from build123d import *

# Parameters (mm, degrees)
SKETCH1_R           = 2
BOSS_EXTRUDE2_DEPTH = 80


with BuildPart() as part:
    # Sketch1 → Boss-Extrude2 (new body)
    with BuildSketch(Plane(origin=(0, 0, 0), x_dir=(1, 0, 0), z_dir=(0, 1, 0))):
        Polygon((-12.5, 5.283121635), (-12.5, -5.283121635), (0, -12.5), (12.5, -5.283121635), (12.5, 5.283121635), (0, 12.5), align=None)
        Circle(SKETCH1_R, mode=Mode.SUBTRACT)
        with BuildLine():
            Line((-1.08, 9.382308546), (-1.08, 3.851441289))
            ThreePointArc((-1.08, 3.851441289), (-2.828427125, 2.828427125), (-3.851441289, 1.08))
            Line((-3.851441289, 1.08), (-10.34, 1.08))
            Line((-10.34, 1.08), (-10.34, 4.036045054))
            Line((-10.34, 4.036045054), (-1.08, 9.382308546))
        make_face(mode=Mode.SUBTRACT)
        with BuildLine():
            Line((1.08, 9.382308546), (1.08, 3.851441289))
            ThreePointArc((1.08, 3.851441289), (2.828427125, 2.828427125), (3.851441289, 1.08))
            Line((3.851441289, 1.08), (10.34, 1.08))
            Line((10.34, 1.08), (10.34, 4.036045054))
            Line((10.34, 4.036045054), (1.08, 9.382308546))
        make_face(mode=Mode.SUBTRACT)
        with BuildLine():
            Line((-10.34, -1.08), (-3.851441289, -1.08))
            ThreePointArc((-3.851441289, -1.08), (-2.828427125, -2.828427125), (-1.08, -3.851441289))
            Line((-1.08, -3.851441289), (-1.08, -9.382308546))
            Line((-1.08, -9.382308546), (-10.34, -4.036045054))
            Line((-10.34, -4.036045054), (-10.34, -1.08))
        make_face(mode=Mode.SUBTRACT)
        with BuildLine():
            Line((1.08, -3.851441289), (1.08, -9.382308546))
            Line((1.08, -9.382308546), (10.34, -4.036045054))
            Line((10.34, -4.036045054), (10.34, -1.08))
            Line((10.34, -1.08), (3.851441289, -1.08))
            ThreePointArc((3.851441289, -1.08), (2.828427125, -2.828427125), (1.08, -3.851441289))
        make_face(mode=Mode.SUBTRACT)
    extrude(amount=BOSS_EXTRUDE2_DEPTH)


solid = part.part
Verification items for the finished model (mm, model axes). A direction names the side the tool comes from. Give positions to 0.01 mm unless a question says otherwise; leave off trailing zeros. Write each loop counter-clockwise with the first axis right and the second up, starting at its lowest first coordinate (ties: lowest second). Pieces come first, ordered by that corner, then holes. Notation, with made-up numbers: M -38,13 L 6,13 A35 cw 6,47 Z; hole C 38.5,9 d6. An arc over 180 degrees is marked long. Write item = value, one per line.
(1) Go/stop test with flat-tipped pins: pin 1 Ø3 at (x, y) = (8.5, 22.5) entering from -Z; pin 2 Ø1.7 at (y, z) = (30, 7) entering from +X; pin 3 Ø5 at (x, y) = (-6, 43) entering from -Z; pin 4 Ø1 at (x, z) = (-4, 3.5) entering from +Y. Record where each tip stops, or that it passes through.
Found:
pin_1 = -8.46
pin_2 = 11
pin_3 = -10.48
pin_4 = through
(2) Sectioned sample at A-A (z = 0). Record the cut outline in (x, y), then the cut area to 3 significant figures.
Found:
outline = M -12.5,0 L -2,0 L -2,80 L -12.5,80 Z; M 2,0 L 12.5,0 L 12.5,80 L 2,80 Z
area = 1,680 mm2
(3) Sectioned sample at C-C (x = 5.5). Record the cut outline in (y, z), then the cut area to 3 significant figures.
Found:
outline = M 0,-9.32 L 80,-9.32 L 80,-6.83 L 0,-6.83 Z; M 0,-1.08 L 80,-1.08 L 80,1.08 L 0,1.08 Z; M 0,6.83 L 80,6.83 L 80,9.32 L 0,9.32 Z
area = 572 mm2
(4) Material ranges on line 1 (X direction, y = 75, z = -0.25); line 2 (Z direction, x = 0, y = 59); line 3 (X direction, y = 41.5, z = 1.75), recorded low to high.
Found:
line_1 = -12.5 to -1.98, 1.98 to 12.5
line_2 = -12.5 to -2, 2 to 12.5
line_3 = -12.5 to -10.34, -3.6 to -0.97, 0.97 to 3.6, 10.34 to 12.5
(5) Draft check along Z on faces 1 (the face through (-6.34, 39.44, 8.84)), 2 (the face through (-2.849, 39.44, 2.808)), 3 (the face through (3, 0, 0)). Enter one of: released by +Z, released by -Z, zero draft, split by the parting line, or undercut.
Found:
face_1 = released by +Z
face_2 = undercut
face_3 = zero draft
(6) Sectioned sample at D-D (z = 6). Record the cut outline in (x, y).
Found:
outline = M -11.26,0 L -6.94,0 L -6.94,80 L -11.26,80 Z; M -1.08,0 L 1.08,0 L 1.08,80 L -1.08,80 Z; M 6.94,0 L 11.26,0 L 11.26,80 L 6.94,80 Z
(7) Sectioned sample at B-B (y = 24.5). Record the cut outline in (x, z), then the cut area to 3 significant figures.
Found:
outline = M -12.5,-5.28 L 0,-12.5 L 12.5,-5.28 L 12.5,5.28 L 0,12.5 L -12.5,5.28 Z; hole M -10.34,-4.04 L -1.08,-9.38 L -1.08,-3.85 A4 cw -3.85,-1.08 L -10.34,-1.08 Z; hole M -10.34,1.08 L -3.85,1.08 A4 cw -1.08,3.85 L -1.08,9.38 L -10.34,4.04 Z; hole C 0,0 d4; hole M 1.08,-9.38 L 10.34,-4.04 L 10.34,-1.08 L 3.85,-1.08 A4 cw 1.08,-3.85 Z; hole M 1.08,3.85 A4 cw 3.85,1.08 L 10.34,1.08 L 10.34,4.04 L 1.08,9.38 Z
area = 244 mm2
(8) Access from +Z, -Z, +X, -X, +Y, -Y to the whole of each face (thin tool, end or side, straight path). Record for faces 4 (the face through (-12.5, 39, 0)), 5 (the face through (7, 39, -1.08)).
Found:
face_4 = +Z, -Z, -X, +Y, -Y
face_5 = +Y, -Y
